CAD build for the part. Positions are in the model's coordinates, mm. A direction names the side the tool comes from. Coordinates: 2 decimals unless noted, no trailing zeros. Loops run counter-clockwise (first coordinate to the right, second up) from the corner with the lowest first, then second, coordinate; pieces in that order, holes last. Notation, with made-up numbers: M 74,-22 L 119,-22 A19 cw 119,6 Z; hole C -7.5,22.25 d7. An arc over 180 degrees is marked long. Answer as a JSON object with one key per item and string values. Group by question number.
```python
from build123d import *

# Parameters (mm, degrees)
SKETCH_W        = 79
SKETCH_H        = 61
SKETCH_W_2      = 73
SKETCH_H_2      = 55
PAD_DEPTH       = 17
SKETCH001_W     = 12.386978
SKETCH001_H     = 11.131831
POCKET_DEPTH    = 3
SKETCH002_W     = 79
SKETCH002_H     = 61
PAD001_DEPTH    = 3
PAD002_DEPTH    = 24
SKETCH004_W     = 48
SKETCH004_H     = 42
POCKET001_DEPTH = 44.001
SKETCH005_R     = 2.6
POCKET002_DEPTH = 65.001
SKETCH006_R     = 2.6
POCKET003_DEPTH = 53.001
SKETCH007_R     = 2.6
POCKET004_DEPTH = 1.5
SKETCH014_R     = 1
POCKET010_DEPTH = 44.001
POCKET013_DEPTH = 1
SKETCH018_W     = 79
SKETCH018_H     = 61
SKETCH018_W_2   = 75
SKETCH018_H_2   = 57
PAD004_DEPTH    = 3
SKETCH027_R     = 2
SKETCH027_R_2   = 1
PAD008_DEPTH    = 4.5
PAD009_DEPTH    = 23
SKETCH032_R     = 1
POCKET018_DEPTH = 19
PAD011_DEPTH    = 0.5


with BuildPart() as part:
    # Sketch → Pad (new body)
    with BuildSketch(Plane.XY):
        Rectangle(SKETCH_W, SKETCH_H)
        Rectangle(SKETCH_W_2, SKETCH_H_2, mode=Mode.SUBTRACT)
    extrude(amount=-PAD_DEPTH)

    # Sketch001 (on Face2 of Pad) → Pocket (cut)
    with BuildSketch(Plane.YZ.offset(39.5)):
        with Locations((11.641985, -11.4340845)):
            Rectangle(SKETCH001_W, SKETCH001_H)
    extrude(amount=-POCKET_DEPTH, mode=Mode.SUBTRACT)

    # Sketch002 (on Face4 of Pocket) → Pad001 (join)
    with BuildSketch(Plane.XY):
        Rectangle(SKETCH002_W, SKETCH002_H)
    extrude(amount=PAD001_DEPTH)

    # Sketch003 (on Face12 of Pad001) → Pad002 (join)
    with BuildSketch(Plane.XY.offset(3)):
        with BuildLine():
            Line((20.5, 22.5), (-20.5, 22.5))
            ThreePointArc((-20.5, 22.5), (-29.0355339059, 26.0355339059), (-25.5, 17.5))
            Line((-25.5, 17.5), (-25.5, -17.5))
            ThreePointArc((-25.5, -17.5), (-29.0355339059, -26.0355339059), (-20.5, -22.5))
            Line((-20.5, -22.5), (20.5, -22.5))
            ThreePointArc((20.5, -22.5), (29.0355339059, -26.0355339059), (25.5, -17.5))
            Line((25.5, -17.5), (25.5, 17.5))
            ThreePointArc((25.5, 17.5), (29.0355339059, 26.0355339059), (20.5, 22.5))
        make_face()
    extrude(amount=PAD002_DEPTH)

    # Sketch004 (on Face27 of Pad002) → Pocket001 (cut, through all)
    with BuildSketch(Plane.XY.offset(27)):
        Rectangle(SKETCH004_W, SKETCH004_H)
    extrude(amount=-POCKET001_DEPTH, mode=Mode.SUBTRACT)

    # Sketch005 (on Face24 of Pocket001) → Pocket002 (cut, through all)
    with BuildSketch(Plane.YZ.offset(25.5)):
        with Locations((-5.105409, 27)):
            Circle(SKETCH005_R)
        with Locations((6.42069, 27)):
            Circle(SKETCH005_R)
    extrude(amount=-POCKET002_DEPTH, mode=Mode.SUBTRACT)

    # Sketch006 (on Face22 of Pocket002) → Pocket003 (cut, through all)
    with BuildSketch(Plane.XZ.offset(22.5)):
        with Locations((-11.5015881496, 27)):
            Circle(SKETCH006_R)
        with Locations((11.491391, 27)):
            Circle(SKETCH006_R)
    extrude(amount=-POCKET003_DEPTH, mode=Mode.SUBTRACT)

    # Sketch007 (on Face18 of Pocket003) → Pocket004 (cut)
    with BuildSketch(Plane(origin=(0, 22.5, 0), x_dir=(-1, 0, 0), z_dir=(0, 1, 0))):
        with Locations((0, 27)):
            Circle(SKETCH007_R)
    extrude(amount=-POCKET004_DEPTH, mode=Mode.SUBTRACT)

    # Sketch014 (on Face34 of Pocket004) → Pocket010 (cut, through all)
    with BuildSketch(Plane.XY.offset(27)):
        with Locations((25.5, 22.5)):
            Circle(SKETCH014_R)
        with Locations((25.5, -22.5)):
            Circle(SKETCH014_R)
        with Locations((-25.5, -22.5)):
            Circle(SKETCH014_R)
        with Locations((-25.5, 22.5)):
            Circle(SKETCH014_R)
    extrude(amount=-POCKET010_DEPTH, mode=Mode.SUBTRACT)

    # Sketch019 (on Face22 of Pocket010) → Pocket013 (cut)
    with BuildSketch(Plane.XZ.offset(22.5)):
        with BuildLine():
            Line((2.8434957673, 7.4753916627), (2.8434957673, 3))
            Line((2.8434957673, 3), (-2.8434957673, 3))
            Line((-2.8434957673, 3), (-2.8434957673, 7.4753916627))
            ThreePointArc((0, 11.483943), (-1.9586480903, 9.8605214945), (-2.8434957673, 7.4753916627))
            ThreePointArc((2.8434957673, 7.4753916627), (1.9586480903, 9.8605214945), (0, 11.483943))
        make_face()
    extrude(amount=-POCKET013_DEPTH, mode=Mode.SUBTRACT)

    # Sketch018 (on Face12 of Pocket010) → Pad004 (join)
    with BuildSketch(Plane.XY.offset(3)):
        Rectangle(SKETCH018_W, SKETCH018_H)
        Rectangle(SKETCH018_W_2, SKETCH018_H_2, mode=Mode.SUBTRACT)
    extrude(amount=PAD004_DEPTH)

    # Sketch027 (on Face21 of Pad004) → Pad008 (join)
    with BuildSketch(Plane(origin=(0, 0, 0), x_dir=(1, 0, 0), z_dir=(0, 0, -1))):
        with Locations((-32.791588, 18.93561)):
            Circle(SKETCH027_R)
        with Locations((-32.791588, 18.93561)):
            Circle(SKETCH027_R_2, mode=Mode.SUBTRACT)
        with Locations((19.386917, 24.113913)):
            Circle(SKETCH027_R)
        with Locations((19.386917, 24.113913)):
            Circle(SKETCH027_R_2, mode=Mode.SUBTRACT)
        with Locations((18.004272, -24.177277)):
            Circle(SKETCH027_R)
        with Locations((18.004272, -24.177277)):
            Circle(SKETCH027_R_2, mode=Mode.SUBTRACT)
        with Locations((-32.796551, -9.026267)):
            Circle(SKETCH027_R)
        with Locations((-32.796551, -9.026267)):
            Circle(SKETCH027_R_2, mode=Mode.SUBTRACT)
    extrude(amount=PAD008_DEPTH)

    # Sketch028 (on Face5 of Pad008) → Pad009 (join)
    with BuildSketch(Plane(origin=(0, 0, -17), x_dir=(1, 0, 0), z_dir=(0, 0, -1))):
        with BuildLine():
            ThreePointArc((39.5, 22.5), (45.1568542495, 36.1568542495), (31.5, 30.5))
            Line((31.5, 30.5), (39.5, 30.5))
            Line((39.5, 30.5), (39.5, 22.5))
        make_face()
        with BuildLine():
            ThreePointArc((-31.5, 30.5), (-45.1568542495, 36.1568542495), (-39.5, 22.5))
            Line((-39.5, 22.5), (-39.5, 30.5))
            Line((-39.5, 30.5), (-31.5, 30.5))
        make_face()
        with BuildLine():
            ThreePointArc((-39.5, -22.5), (-45.1568542495, -36.1568542495), (-31.5, -30.5))
            Line((-31.5, -30.5), (-39.5, -30.5))
            Line((-39.5, -30.5), (-39.5, -22.5))
        make_face()
        with BuildLine():
            ThreePointArc((31.5, -30.5), (45.1568542495, -36.1568542495), (39.5, -22.5))
            Line((39.5, -22.5), (39.5, -30.5))
            Line((39.5, -30.5), (31.5, -30.5))
        make_face()
    extrude(amount=-PAD009_DEPTH)

    # Sketch032 (on Face12 of Pad009) → Pocket018 (cut)
    with BuildSketch(Plane(origin=(0, 0, -17), x_dir=(1, 0, 0), z_dir=(0, 0, -1))):
        with Locations((39.5, 30.5)):
            Circle(SKETCH032_R)
        with Locations((39.5, -30.5)):
            Circle(SKETCH032_R)
        with Locations((-39.5, 30.5)):
            Circle(SKETCH032_R)
        with Locations((-39.5, -30.5)):
            Circle(SKETCH032_R)
    extrude(amount=-POCKET018_DEPTH, mode=Mode.SUBTRACT)

    # Sketch033 (on Face89 of Pocket018) → Pad011 (join)
    with BuildSketch(Plane.XZ.offset(22.5)):
        Polygon((-10.2987765, 19.4466314572), (-6.2987765, 19.4466314572), (-6.2987765, 7.4466314572), (-8.2987765, 9.4466314572), (-10.2987765, 7.4466314572), align=None)
        Polygon((6.2987765, 19.4453464572), (10.2987765, 19.4453464572), (10.2987765, 7.4453464572), (8.2987765, 9.4453464572), (6.2987765, 7.4453464572), align=None)
    extrude(amount=PAD011_DEPTH)


solid = part.part
```
Item 1: Slice it at B-B, the plane z = 22.5. Write the cut outline in (x, y).
Item 2: Drill centre lines: L1, parallel to X at y = -16, z = 18; L2, parallel to X at y = -17, z = 5.5; L3, parallel to X at y = -3, z = -9. Where is each one in solid material? Low to high. Write a range as from..to.
Item 3: Slice it at D-D, the plane z = -2. Count the separate pieces of the cut face and the enclosed holes in it, then the cut area to 3 significant figures.
Item 4: Tool access for faces 1 (the cylindrical face through (2, -22, 9.8)), 2 (the flat face through (38, 5.448, -12)), 3 (the flat face through (8, -23, 14)), 4 (the flat face through (-25, 0, 0)), 5 (the cylindrical face through (28.92, -26.15, 14.83)): list every direction of +Z, -Z, +X, -X, +Y, -Y with a clear straight run to the whole face (end or side of a thin tool).
Item 5: Slice it at A-A, the plane z = -10. Write the cut outline in (x, y), then the cut area to 3 significant figures.
Item 6: Pin check, flat tips, straight feed: pin 1 (5 mm diameter, centred on y = -22, z = -11.5, fed in from +X); pin 2 (8 mm diameter, centred on x = -10.5, z = 10.5, fed in from +Y); pin 3 (3 mm diameter, centred on x = -32.5, y = -18.5, fed in from -Z). Stop position of each tip, or through.
Item 7: Pull direction X, two halves, no side cores. Call faces 6 (the cylindrical face through (-24.7, -5.2, 24.4)), 7 (the flat face through (-1, 28.5, 4)): released by +X, released by -X, zero draft, split by the parting line, or undercut.
Item 8: Slice it at C-C, the plane x = -22. Write the cut outline in (y, z).
Computed:
{
 "1": {"outline": "M -25.5,-17.5 A5 ccw long -20.5,-22.5 L 20.5,-22.5 A5 ccw long 25.5,-17.5 L 25.5,17.5 A5 ccw long 20.5,22.5 L -20.5,22.5 A5 ccw long -25.5,17.5 Z; hole C -25.5,-22.5 d2; hole C -25.5,22.5 d2; hole M -24,-21 L 24,-21 L 24,21 L -24,21 Z; hole C 25.5,-22.5 d2; hole C 25.5,22.5 d2"},
 "2": {"L1": "-25.5..-24, 24..25.5", "L2": "-39.5..-37.5, -25.5..-24, 24..25.5, 37.5..39.5", "L3": "-39.5..-36.5, 36.5..39.5"},
 "3": {"separate pieces": "5", "enclosed holes": "9", "area": "1,430 mm2"},
 "4": {"face 1": "-Y", "face 2": "-Z, +X", "face 3": "+Z, -Y", "face 4": "-Z", "face 5": "+Z"},
 "5": {"outline": "M -39.5,-22.5 A8 ccw long -31.5,-30.5 L 31.5,-30.5 A8 ccw long 39.5,-22.5 L 39.5,5.45 L 36.5,5.45 L 36.5,-27.5 L -36.5,-27.5 L -36.5,27.5 L 36.5,27.5 L 36.5,17.84 L 39.5,17.84 L 39.5,22.5 A8 ccw long 31.5,30.5 L -31.5,30.5 A8 ccw long -39.5,22.5 Z; hole C -39.5,-30.5 d2; hole C -39.5,30.5 d2; hole C 39.5,-30.5 d2; hole C 39.5,30.5 d2", "area": "1,360 mm2"},
 "6": {"pin 1": "x = 44.79", "pin 2": "y = 22.5", "pin 3": "z = -4.5"},
 "7": {"face 6": "zero draft", "face 7": "undercut"},
 "8": {"outline": "M -30.5,-17 L -27.5,-17 L -27.5,0 L -21,0 L -21,27 L -26.07,27 L -26.07,3 L -28.5,3 L -28.5,6 L -30.5,6 Z; M 21,0 L 27.5,0 L 27.5,-17 L 30.5,-17 L 30.5,6 L 28.5,6 L 28.5,3 L 26.07,3 L 26.07,27 L 21,27 Z"}
}
